Can you work these out from the model? Positions are in its coordinate system, mm. Give positions to 0.01 mm unless a question says otherwise; leave off trailing zeros. Loops run counter-clockwise (first coordinate to the right, second up) from the corner with the lowest first, then second, coordinate; pieces in that order, holes last. Notation, with made-up numbers: M 19,4.25 L 36,4.25 A27 ccw 36,23.25 Z; hole C 53,60.5 d4. An arc over 180 degrees is marked long. Answer as a JSON object with one key per item and string values.
```python
from build123d import *

# Parameters (mm, degrees)
BOSS_EXTRUDE1_DEPTH = 3
SKETCH6_R           = 1
CUT_EXTRUDE1_DEPTH  = 3
CHAMFER1_SIZE       = 1.25


with BuildPart() as part:
    # Sketch1 → Boss-Extrude1 (new body)
    with BuildSketch(Plane(origin=(0, 0, 0), x_dir=(0, 1, 0), z_dir=(0, 0, 1))):
        with BuildLine():
            Line((-35, 4.4), (35, 4.4))
            ThreePointArc((35, 4.4), (39.4, 0), (35, -4.4))
            Line((35, -4.4), (-35, -4.4))
            ThreePointArc((-35, -4.4), (-39.4, 0), (-35, 4.4))
        make_face()
    extrude(amount=BOSS_EXTRUDE1_DEPTH)

    # Sketch6 → Cut-Extrude1 (cut)
    with BuildSketch(Plane.XY.offset(3)):
        with Locations((0, 35)):
            Circle(SKETCH6_R)
        with Locations((0, -35)):
            Circle(SKETCH6_R)
        Circle(SKETCH6_R)
    extrude(amount=-CUT_EXTRUDE1_DEPTH, mode=Mode.SUBTRACT)

    # Chamfer1
    chamfer1_edges = [part.edges().sort_by_distance(p)[0] for p in [
        (-1, 35, 0),
        (-1, -35, 0),
        (-1, 0, 0),
    ]]
    chamfer(chamfer1_edges, length=CHAMFER1_SIZE)


solid = part.part
```
1) Suppose I cut it at B-B, the plane z = 2.4. Write out the boundary of the cut face in (x, y).
Answer list:
{"outline": "M -4.4,-35 A4.4 ccw 4.4,-35 L 4.4,35 A4.4 ccw -4.4,35 Z; hole C 0,-35 d2; hole C 0,0 d2; hole C 0,35 d2"}
2) Suppose I cut it at C-C, the plane y = 0. Write out the boundary of the cut face in (x, z).
Answer list:
{"outline": "M -4.4,0 L -2.25,0 L -1,1.25 L -1,3 L -4.4,3 Z; M 1,1.25 L 2.25,0 L 4.4,0 L 4.4,3 L 1,3 Z"}
3) Suppose I cut it at D-D, the plane x = 3. Write out the boundary of the cut face in (y, z).
Answer list:
{"outline": "M -38.22,0 L 38.22,0 L 38.22,3 L -38.22,3 Z"}
4) Please list where these lines run through material, in increasing order: line 1 along Y through (x, z) = (0, 1.75); line 2 along Y through (x, z) = (-0.5, 2.2); line 3 along Y through (x, z) = (-3.5, 0.3). Write a range as from..to.
Answer list:
{"line 1": "-39.4..-36, -34..-1, 1..34, 36..39.4", "line 2": "-39.37..-35.87, -34.13..-0.87, 0.87..34.13, 35.87..39.37", "line 3": "-37.67..37.67"}
5) Suppose I cut it at A-A, the plane x = 0. Write out the boundary of the cut face in (y, z), and give its area (3 significant figures).
Answer list:
{"outline": "M -39.4,0 L -37.25,0 L -36,1.25 L -36,3 L -39.4,3 Z; M -34,1.25 L -32.75,0 L -2.25,0 L -1,1.25 L -1,3 L -34,3 Z; M 1,1.25 L 2.25,0 L 32.75,0 L 34,1.25 L 34,3 L 1,3 Z; M 36,1.25 L 37.25,0 L 39.4,0 L 39.4,3 L 36,3 Z", "area": "214 mm^2"}
6) If we mould it in two halves opening along Y, with no side actions, what happens to faces 1 (the cylindrical face through (0, -34, 2)), 2 (the cylindrical face through (0, 36, 2)), 3 (the flat face through (-3, 1, 0)), 4 (the cylindrical face through (0.1, -39.4, 1.5))? For each: +Y half, -Y half, draft (parallel to the pull), parting line (faces both ways), or undercut.
Answer list:
{"face 1": "undercut", "face 2": "undercut", "face 3": "draft", "face 4": "-Y half"}
7) Will these pins go through, and if not, where does the flat tip stop? pin 1 Ø1.5 at (x, z) = (-1.5, 2) entering from -Y; pin 2 Ø1.5 at (x, z) = (-1, 0.5) entering from +Y; pin 3 Ø3 at (x, y) = (0, 35) entering from +Z.
Answer list:
{"pin 1": "y = -39.34", "pin 2": "y = 39.39", "pin 3": "z = 3"}
